Could you check a few things on this model? Use its own coordinates, in mm. Coordinates: 2 decimals unless noted, no trailing zeros. Loops run counter-clockwise (first coordinate to the right, second up) from the corner with the lowest first, then second, coordinate; pieces in that order, holes last. Notation, with made-up numbers: M -33.75,21.5 L -28.75,21.5 A21 ccw -28.75,33.5 Z; hole C 60,73 d5. An arc over 180 degrees is marked long. Write each question's results on one line, items separated by ' | '.
```python
from build123d import *

# Parameters (mm, degrees)
SKETCH1_R           = 3.175
BOSS_EXTRUDE1_DEPTH = 9


with BuildPart() as part:
    # Sketch1 → Boss-Extrude1 (new body)
    with BuildSketch(Plane.XY):
        with BuildLine():
            Line((-8.032782944, 13.219871482), (-8.032782944, -13.219871482))
            Line((-8.032782944, -13.219871482), (8.032782944, -13.219871482))
            Line((8.032782944, -13.219871482), (8.032782944, 13.219871482))
            ThreePointArc((8.032782944, 13.219871482), (5.680035292, 18.899906774), (0, 21.252654427))
            ThreePointArc((0, 21.252654427), (-5.680035292, 18.899906774), (-8.032782944, 13.219871482))
        make_face()
        with Locations((0, 13.219871482)):
            Circle(SKETCH1_R, mode=Mode.SUBTRACT)
    extrude(amount=BOSS_EXTRUDE1_DEPTH)


solid = part.part
```
(1) Imagine slicing it at C-C, the plane x = -6.5. List the corners of the cut face in (y, z) for me.
Reported:
outline: M -13.22,0 L 17.94,0 L 17.94,9 L -13.22,9 Z
(2) If we mould it in two halves opening along X, with no side actions, what happens to faces 1 (the flat face through (-8.033, 0, 4)), 2 (the flat face through (8.033, 0, 4)), 3 (the flat face through (0, 4, 0)), 4 (the cylindrical face through (-0.69, 10.12, 4.44))? For each: released by +X, released by -X, zero draft, split by the parting line, or undercut.
Reported:
face 1: released by -X | face 2: released by +X | face 3: zero draft | face 4: undercut
(3) Imagine slicing it at D-D, the plane x = 6.75. List the corners of the cut face in (y, z) for me.
Reported:
outline: M -13.22,0 L 17.57,0 L 17.57,9 L -13.22,9 Z
(4) Please list where these lines run through material, in increasing order: probe 1 along X at (y, z) = (14.5, 0.5); probe 2 along Y at (x, z) = (2.75, 1.25); probe 3 along Y at (x, z) = (1, 3.5). Write a range as from..to.
Reported:
probe 1: x = -7.93..-2.91, 2.91..7.93 | probe 2: y = -13.22..11.63, 14.81..20.77 | probe 3: y = -13.22..10.21, 16.23..21.19
(5) Imagine slicing it at B-B, the plane y = 11. List the corners of the cut face in (x, z) for me.
Reported:
outline: M -8.03,0 L -2.27,0 L -2.27,9 L -8.03,9 Z; M 2.27,0 L 8.03,0 L 8.03,9 L 2.27,9 Z
(6) Imagine slicing it at A-A, the plane x = 1. List the corners of the cut face in (y, z) for me, and give its area (3 significant figures).
Reported:
outline: M -13.22,0 L 10.21,0 L 10.21,9 L -13.22,9 Z; M 16.23,0 L 21.19,0 L 21.19,9 L 16.23,9 Z | area: 255 mm2
